Can you work these out from the model? Positions are in its coordinate system, mm. Round coordinates to 2 decimals unless told otherwise and drop trailing zeros. Write each loop counter-clockwise with the first axis right and the second up, starting at its lowest first coordinate (ties: lowest second). Pieces come first, ordered by that corner, then holes.
Q1. Please list where these lines run through material, in increasing order: line 1 along X through (y, z) = (0.7, 19); line 2 along X through (y, z) = (1.2, 26.5); line 3 along Z through (x, y) = (168.9, 1.55).
Q2. If we section it at A-A (z = 34.5): Please give me the cut outline in (x, y).
Q3. I'm going to push flat-ended pins straight in: pin 1 Ø6 at (x, z) = (168.9, 26.5) entering from +Y; pin 2 Ø3 at (x, z) = (111.1, 26.5) entering from +Y. Where does each tip first touch, or does it pass through?
from build123d import *

# Parameters (mm, degrees)
BOSS_EXTRUDE1_DEPTH   = 3
F_6_CLEARANCE_HOLE1_D = 3.7973
SKETCH4_R             = 0.25
CUT_EXTRUDE1_DEPTH    = 10


with BuildPart() as part:
    # Sketch1 → Boss-Extrude1 (new body)
    with BuildSketch(Plane(origin=(0, 0, 0), x_dir=(1, 0, 0), z_dir=(0, 1, 0))):
        with BuildLine():
            Line((10, 0), (270, 0))
            ThreePointArc((270, 0), (277.071067812, -2.928932188), (280, -10))
            Line((280, -10), (280, -28))
            ThreePointArc((280, -28), (277.071067812, -35.071067812), (270, -38))
            Line((270, -38), (10, -38))
            ThreePointArc((10, -38), (2.928932188, -35.071067812), (0, -28))
            Line((0, -28), (0, -10))
            ThreePointArc((0, -10), (2.928932188, -2.928932188), (10, 0))
        make_face()
    extrude(amount=BOSS_EXTRUDE1_DEPTH)

    # #6 Clearance Hole1 (through all)
    with Locations(Plane(origin=(0, 3, 0), x_dir=(1, 0, 0), z_dir=(0, 1, 0))):
        with Locations((111.1, -11.5), (111.1, -26.5), (168.9, -26.5), (168.9, -11.5)):
            Hole(F_6_CLEARANCE_HOLE1_D / 2)

    # Sketch4 → Cut-Extrude1 (cut)
    with BuildSketch(Plane(origin=(0, 3, 0), x_dir=(1, 0, 0), z_dir=(0, 1, 0))):
        with Locations(Location((70, -19, 0), (0, 0, 270))):
            Circle(SKETCH4_R)
        with Locations(Location((140, -19, 0), (0, 0, 270))):
            Circle(SKETCH4_R)
        with Locations(Location((210, -19, 0), (0, 0, 270))):
            Circle(SKETCH4_R)
    extrude(amount=-CUT_EXTRUDE1_DEPTH, mode=Mode.SUBTRACT)


solid = part.part
A:
1. line 1: x = 0 to 69.75, 70.25 to 139.75, 140.25 to 209.75, 210.25 to 280
1. line 2: x = 0 to 109.2, 113 to 167, 170.8 to 280
1. line 3: z = 0 to 9.6, 13.4 to 24.6, 28.4 to 38
2. outline: (2.4, 0) - (277.6, 0) - (277.6, 3) - (2.4, 3) - close
3. pin 1: stops at y = 3
3. pin 2: passes through
